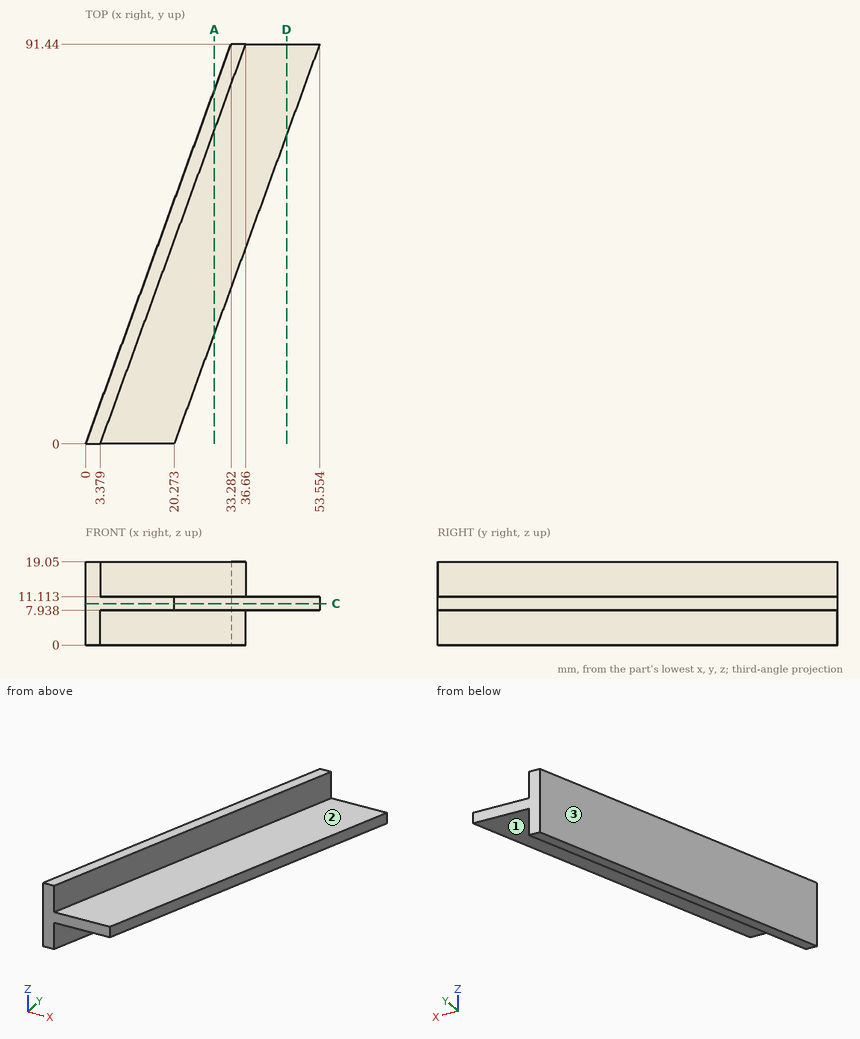
Print and shaded views of the part. All mm, measured from the part's lowest x, y and z. A direction names the side the tool comes from. Round coordinates to 2 decimals unless told otherwise and drop trailing zeros. Loops run counter-clockwise (first coordinate to the right, second up) from the corner with the lowest first, then second, coordinate; pieces in that order, holes last. Notation, with made-up numbers: M 12,42 L 19,42 A23 cw 19,67 Z; hole C 55,-34 d3. An arc over 180 degrees is marked long. One line per question, with ' | ' between items.
1) Band-saw the part on A-A (x = 29.5). Give the cut face in (y, z).
Solved:
outline: M 25.35,7.94 L 71.77,7.94 L 71.77,0 L 81.05,0 L 81.05,19.05 L 71.77,19.05 L 71.77,11.11 L 25.35,11.11 Z
2) 3-axis set-ups, long thin cutter, end or side, ignore diameter. For the marked faces 1, 2 and 3: which of +Z, -Z, +X, -X, +Y, -Y reach the whole face in a straight line?
Solved:
face 1: -Z, +X, -Y | face 2: +Z, +X, -Y | face 3: +Z, -Z, -X, +Y
3) Band-saw the part on D-D (x = 46). Give the cut face in (y, z) (1 decimal).
Solved:
outline: M 70.7,7.9 L 91.4,7.9 L 91.4,11.1 L 70.7,11.1 Z
4) Drill centre lines: line 1 along Z through (x, y) = (30, 60.5); line 2 along X through (y, z) = (22, 17.5) (1 decimal); line 3 along X through (y, z) = (32, 12.75) (1 decimal). Where is each one in solid material? Low to high.
Solved:
line 1: z = 7.94 to 11.11 | line 2: x = 8 to 11.4 | line 3: x = 11.6 to 15
5) Band-saw the part on C-C (z = 9.5). Give the cut face in (x, y) (1 decimal).
Solved:
outline: M 0,0 L 20.3,0 L 53.6,91.4 L 33.3,91.4 Z
6) Flat gauge pins, fed straight in: pin 1 (10 mm diameter, centred on y = 16, z = 15.5, fed in from +X); pin 2 (4 mm diameter, centred on y = 53, z = 2, fed in from +X); pin 3 (10 mm diameter, centred on y = 70, z = 12.5, fed in from +X). Where does each tip first touch, or does it go through?
Solved:
pin 1: stops at x = 26.97 | pin 2: stops at x = 23.4 | pin 3: stops at x = 47.5
